Part model, mm, in its own coordinate system. A direction names the side the tool comes from. Round coordinates to 2 decimals unless told otherwise and drop trailing zeros. Write each loop counter-clockwise with the first axis right and the second up, starting at its lowest first coordinate (ties: lowest second). Pieces come first, ordered by that corner, then holes.
1) Which spindle directions (+Z, -Z, +X, -X, +Y, -Y) get a long thin tool onto all of the face, cutting with end or side? Do faces 1 (the flat face through (-67, 2, -25)), 2 (the flat face through (12, 2, 34)), 3 (the flat face through (-1, 9, 4)). Say none if no direction does.
2) Saw through at D-D on x = -55.5. Write the cut outline in (y, z), and give its area (3 significant figures).
3) Drill centre lines: L1, parallel to X at y = 1.05, z = 52; L2, parallel to Z at x = 9.5, y = 7.25; L3, parallel to X at y = 1.3, z = 36.5. Where is each one in solid material? Low to high.
4) Pull direction X, two halves, no side cores. Call faces 4 (the flat face through (-1, 11, -2)), 5 (the cylindrical face through (45, 2, -34)), 6 (the flat face through (-25, 2, 78)): +X half, -X half, draft (parallel to the pull), parting line (faces both ways), or undercut.
5) Saw through at B-B on y = 7.5. Write the cut outline in (x, z).
6) Saw through at C-C on x = 50. Write the cut outline in (y, z), and give its area (3 significant figures).
7) Flat gauge pins, fed straight in: pin 1 (8 mm diameter, centred on y = 5, z = -31.5, fed in from -X); pin 2 (3 mm diameter, centred on x = -40.5, y = 2.5, fed in from -Z); pin 3 (4.5 mm diameter, centred on x = -38, y = 2, fed in from +Z); pin 4 (5 mm diameter, centred on x = 46, z = 36.5, fed in from -Y). Where does each tip first touch, or does it go through?
8) Saw through at A-A on z = -34. Write the cut outline in (x, y).
```python
from build123d import *

# Parameters (mm, degrees)
BOSS_EXTRUDE1_DEPTH = 4
SKETCH4_W           = 130
SKETCH4_H           = 4
BOSS_EXTRUDE2_DEPTH = 10
SKETCH5_W           = 130
SKETCH5_H           = 4
BOSS_EXTRUDE3_DEPTH = 7
SKETCH6_W           = 130
SKETCH6_H           = 4
BOSS_EXTRUDE4_DEPTH = 10
SKETCH8_W           = 130
SKETCH8_H           = 4
BOSS_EXTRUDE5_DEPTH = 7
CUT_EXTRUDE1_DEPTH  = 107.117859006
CHAMFER2_SIZE       = 4
CHAMFER3_SIZE       = 4
CUT_EXTRUDE3_DEPTH  = 107.117859006
SKETCH12_R          = 1.5
CUT_EXTRUDE4_DEPTH  = 107.117859006
SKETCH13_R          = 6.5
CUT_EXTRUDE5_DEPTH  = 107.117859006
SKETCH14_R          = 4
CUT_EXTRUDE6_DEPTH  = 107.117859006
CUT_EXTRUDE7_DEPTH  = 10


with BuildPart() as part:
    # Sketch3 → Boss-Extrude1 (new body)
    with BuildSketch(Plane(origin=(0, 0, 0), x_dir=(1, 0, 0), z_dir=(0, 1, 0))):
        Polygon((-25, 80), (25, 80), (25, 76), (65, 76), (65, 25), (69, 25), (69, -25), (65, -25), (65, -76), (25, -76), (25, -80), (-25, -80), (-25, -76), (-65, -76), (-65, -25), (-69, -25), (-69, 25), (-65, 25), (-65, 76), (-25, 76), align=None)
    extrude(amount=BOSS_EXTRUDE1_DEPTH)

    # Sketch4 → Boss-Extrude2 (add)
    with BuildSketch(Plane(origin=(0, 4, 0), x_dir=(1, 0, 0), z_dir=(0, 1, 0))):
        with Locations((0, -74)):
            Rectangle(SKETCH4_W, SKETCH4_H)
    extrude(amount=BOSS_EXTRUDE2_DEPTH)

    # Sketch5 → Boss-Extrude3 (add)
    with BuildSketch(Plane(origin=(0, 4, 0), x_dir=(1, 0, 0), z_dir=(0, 1, 0))):
        with Locations((0, -66)):
            Rectangle(SKETCH5_W, SKETCH5_H)
    extrude(amount=BOSS_EXTRUDE3_DEPTH)

    # Sketch6 → Boss-Extrude4 (add)
    with BuildSketch(Plane(origin=(0, 4, 0), x_dir=(1, 0, 0), z_dir=(0, 1, 0))):
        with Locations((0, -6)):
            Rectangle(SKETCH6_W, SKETCH6_H)
    extrude(amount=BOSS_EXTRUDE4_DEPTH)

    # Sketch8 → Boss-Extrude5 (add)
    with BuildSketch(Plane(origin=(0, 4, 0), x_dir=(1, 0, 0), z_dir=(0, 1, 0))):
        with Locations((0, 2)):
            Rectangle(SKETCH8_W, SKETCH8_H)
    extrude(amount=BOSS_EXTRUDE5_DEPTH)

    # Sketch9 → Cut-Extrude1 (cut, through all)
    with BuildSketch(Plane(origin=(0, 4, 0), x_dir=(1, 0, 0), z_dir=(0, 1, 0))):
        Polygon((-21.999983798, -49.3), (-31.999983798, -49.3), (-31.999983798, -42.3), (-40, -42.3), (-40, -31.3), (-35.999983798, -31.3), (-35.999983798, -26.3), (-17.999983798, -26.3), (-17.999983798, -31.3), (-14, -31.311384755), (-14, -42.288615245), (-22, -42.3), align=None)
    extrude(amount=-CUT_EXTRUDE1_DEPTH, mode=Mode.SUBTRACT)

    # Chamfer2
    chamfer2_edges = [part.edges().sort_by_distance(p)[0] for p in [
        (-40, 4, 36.8),
    ]]
    chamfer(chamfer2_edges, length=CHAMFER2_SIZE - 0.0001)  # a hair under: the kernel refuses the full size

    # Chamfer3
    chamfer3_edges = [part.edges().sort_by_distance(p)[0] for p in [
        (-14, 4, 36.8),
    ]]
    chamfer(chamfer3_edges, length=CHAMFER3_SIZE - 0.0001)  # a hair under: the kernel refuses the full size

    # Sketch11 → Cut-Extrude3 (cut, through all)
    with BuildSketch(Plane(origin=(0, 4, 0), x_dir=(1, 0, 0), z_dir=(0, 1, 0))):
        Polygon((12, -27.5), (40, -27.5), (40, -40.5), (34, -46.5), (18, -46.5), (12, -40.5), align=None)
    extrude(amount=-CUT_EXTRUDE3_DEPTH, mode=Mode.SUBTRACT)

    # Sketch12 → Cut-Extrude4 (cut, through all)
    with BuildSketch(Plane(origin=(0, 4, 0), x_dir=(1, 0, 0), z_dir=(0, 1, 0))):
        with Locations(Location((6, -36.5, 0), (0, 0, 270))):
            Circle(SKETCH12_R)
        with Locations(Location((46, -36.5, 0), (0, 0, 270))):
            Circle(SKETCH12_R)
    extrude(amount=-CUT_EXTRUDE4_DEPTH, mode=Mode.SUBTRACT)

    # Sketch13 → Cut-Extrude5 (cut, through all)
    with BuildSketch(Plane(origin=(0, 4, 0), x_dir=(1, 0, 0), z_dir=(0, 1, 0))):
        with Locations(Location((50, -52, 0), (0, 0, 270))):
            Circle(SKETCH13_R)
    extrude(amount=-CUT_EXTRUDE5_DEPTH, mode=Mode.SUBTRACT)

    # Sketch14 → Cut-Extrude6 (cut, through all)
    with BuildSketch(Plane(origin=(0, 4, 0), x_dir=(1, 0, 0), z_dir=(0, 1, 0))):
        with Locations(Location((0, -52, 0), (0, 0, 270))):
            Circle(SKETCH14_R)
    extrude(amount=-CUT_EXTRUDE6_DEPTH, mode=Mode.SUBTRACT)

    # Sketch15 → Cut-Extrude7 (cut)
    with BuildSketch(Plane.XZ):
        with BuildLine():
            Line((-9, -25), (36, -25))
            ThreePointArc((36, -25), (45, -34), (36, -43))
            Line((36, -43), (-9, -43))
            ThreePointArc((-9, -43), (-18, -34), (-9, -25))
        make_face()
    extrude(amount=-CUT_EXTRUDE7_DEPTH, mode=Mode.SUBTRACT)


solid = part.part
```
Completed:
1. face 1: -Z, -X, +Y, -Y
1. face 2: +Y, -Y
1. face 3: +X, -X, +Y
2. outline: (0, -76) - (4, -76) - (4, -4) - (11, -4) - (11, 0) - (4, 0) - (4, 4) - (14, 4) - (14, 8) - (4, 8) - (4, 64) - (11, 64) - (11, 68) - (4, 68) - (4, 72) - (14, 72) - (14, 76) - (0, 76) - close
2. area: 744 mm2
3. L1: x = -65 to -4, 4 to 43.5, 56.5 to 65
3. L2: z = -4 to 0, 4 to 8, 64 to 68, 72 to 76
3. L3: x = -65 to -41.3, -12.7 to 4.5, 7.5 to 12, 40 to 44.5, 47.5 to 65
4. face 4: draft
4. face 5: undercut
4. face 6: -X half
5. outline: (-65, -4) - (65, -4) - (65, 0) - (-65, 0) - close; (-65, 4) - (65, 4) - (65, 8) - (-65, 8) - close; (-65, 64) - (65, 64) - (65, 68) - (-65, 68) - close; (-65, 72) - (65, 72) - (65, 76) - (-65, 76) - close
6. outline: (0, -76) - (4, -76) - (4, -4) - (11, -4) - (11, 0) - (4, 0) - (4, 4) - (14, 4) - (14, 8) - (4, 8) - (4, 45.5) - (0, 45.5) - close; (0, 58.5) - (4, 58.5) - (4, 64) - (11, 64) - (11, 68) - (4, 68) - (4, 72) - (14, 72) - (14, 76) - (0, 76) - close
6. area: 692 mm2
7. pin 1: stops at x = -65
7. pin 2: stops at z = -76
7. pin 3: stops at z = 76
7. pin 4: stops at y = 0
8. outline: (-65, 0) - (-18, 0) - (-18, 4) - (-65, 4) - close; (45, 0) - (65, 0) - (65, 4) - (45, 4) - close
